Source: three-view drawing plus pictorial views. Frame: mm from the lowest corner of the part. Give positions to 0.01 mm unless a question says otherwise; leave off trailing zeros. Order: outer loops, then holes, each group sorted by start corner. A loop starts at its lowest first (then second) coordinate and runs counter-clockwise, first axis right, second up. Notation, with made-up numbers: (-13.75, -12) -> (7.25, -12) arc R10 cw to (7.25, 5) -> close; hole circle Ø3 at (-0.75, -33). An arc over 180 degrees is marked (long way). Answer in a Markdown table with one row per item. Add a question column.
Q1. Cut plane D-D on y = 4.9. Return the cut outline in (x, z), and give its area (3 significant figures).
Q2. Contact query for flat-ended pins moving along their axis: P1, Ø4.5, axis at x = 6.35, y = 159.84, coming from the +Z side; P2, Ø1.6, axis at y = 83, z = 3, coming from the -X side; P3, Ø1, axis at x = 8.5, z = 3, coming from the -Y side. Output: stop coordinate, or through.
Q3. Line query: line 1 along Y through (x, z) = (163.83, 1.25); line 2 along Y through (x, z) = (6.35, 1.25); line 3 along X through (y, z) = (159.84, 1). Output: solid intervals per line, ascending. Write a range as from..to.
Q4. Cut plane A-A on z = 2.6. Return the cut outline in (x, y).
Q5. Cut plane C-C on x = 163.83. Return the cut outline in (y, z), and give its area (3 significant figures).
Q6. Cut plane B-B on y = 136.98. Return the cut outline in (x, z).
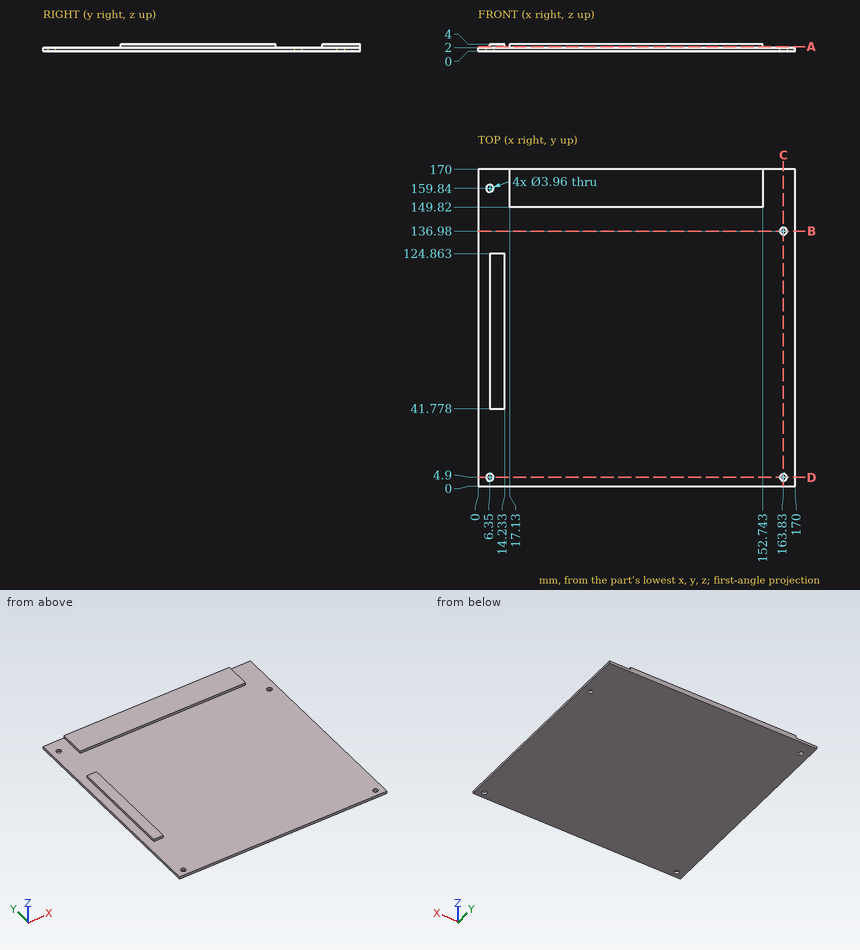
Completed:
| question | item | result |
|---|---|---|
| 1 | outline | (0, 0) -> (4.37, 0) -> (4.37, 2) -> (0, 2) -> close; (8.33, 0) -> (161.85, 0) -> (161.85, 2) -> (8.33, 2) -> close; (165.81, 0) -> (170, 0) -> (170, 2) -> (165.81, 2) -> close |
| 1 | area | 324 mm² |
| 2 | P1 | stops at z = 2 |
| 2 | P2 | stops at x = 6.35 |
| 2 | P3 | stops at y = 41.78 |
| 3 | line 1 | y = 0..2.92, 6.88..135, 138.96..170 |
| 3 | line 2 | y = 0..2.92, 6.88..157.86, 161.82..170 |
| 3 | line 3 | x = 0..4.37, 8.33..170 |
| 4 | outline | (6.35, 41.78) -> (14.23, 41.78) -> (14.23, 124.86) -> (6.35, 124.86) -> close; (17.13, 149.82) -> (152.74, 149.82) -> (152.74, 170) -> (17.13, 170) -> close |
| 5 | outline | (0, 0) -> (2.92, 0) -> (2.92, 2) -> (0, 2) -> close; (6.88, 0) -> (135, 0) -> (135, 2) -> (6.88, 2) -> close; (138.96, 0) -> (170, 0) -> (170, 2) -> (138.96, 2) -> close |
| 5 | area | 324 mm² |
| 6 | outline | (0, 0) -> (161.85, 0) -> (161.85, 2) -> (0, 2) -> close; (165.81, 0) -> (170, 0) -> (170, 2) -> (165.81, 2) -> close |
